The listing builds one solid part. Answer for the finished solid, in the listing's coordinates (mm). A direction names the side the tool comes from. Give positions to 0.01 mm unless a question says otherwise; leave off trailing zeros. Order: outer loops, then holes, each group sorted by start corner. A loop starts at its lowest first (then second) coordinate and runs counter-clockwise, first axis right, second up. Notation, with made-up numbers: M 5,15 L 14,15 A28 cw 14,52 Z; hole C -14,-24.75 d6. An arc over 180 degrees is marked long. Answer as a JSON object with one key per item and string values. Group by question number.
```python
from build123d import *

# Parameters (mm, degrees)
F1_DEPTH = 63.5
F2_DEPTH = 25.4
F3_DEPTH = 15.875


with BuildPart() as f1:
    # F0 (on Front) → F1 (new body, symmetric)
    with BuildSketch(Plane.XZ):
        Polygon((41.275, -9.525), (41.275, 9.525), (22.225, 9.525), (-41.275, 9.525), (-41.275, -9.525), align=None)
    extrude(amount=F1_DEPTH, both=True)

    # F0 (on Front) → F2 (join, symmetric)
    with BuildSketch(Plane.XZ):
        Polygon((41.275, -9.525), (41.275, 9.525), (22.225, 9.525), (-41.275, 9.525), (-41.275, -9.525), align=None)
        with BuildLine():
            Line((22.225, 9.525), (41.275, 9.525))
            Line((41.275, 9.525), (41.275, 36.094566609))
            ThreePointArc((41.275, 36.094566609), (37.2701177009, 42.5355625854), (35.2519640423, 49.8466888466))
            add(Edge.make_bspline(
                [(22.225, 41.2858579773), (27.1473848913, 43.2390175142), (31.5927512489, 45.8874426384), (35.2519640423, 49.8466888466)],
                knots=[68.7075286576, 68.7075286576, 68.7075286576, 68.7075286576, 85.3888938388, 85.3888938388, 85.3888938388, 85.3888938388], degree=3))
            Line((22.225, 41.2858579773), (22.225, 9.525))
        make_face()
        with BuildLine():
            Line((-41.275, 9.525), (22.225, 9.525))
            Line((22.225, 9.525), (22.225, 41.2858579773))
            add(Edge.make_bspline(
                [(-41.275, 9.525), (-26.416290782, 36.991388499), (1.9505861672, 33.2411468041), (22.225, 41.2858579773)],
                knots=[0, 0, 0, 0, 68.7075286576, 68.7075286576, 68.7075286576, 68.7075286576], degree=3))
        make_face()
        with BuildLine():
            ThreePointArc((35.2519640423, 49.8466888466), (37.2701177009, 42.5355625854), (41.275, 36.094566609))
            Line((41.275, 36.094566609), (41.275, 59.3244851528))
            add(Edge.make_bspline(
                [(35.2519640423, 49.8466888466), (37.6153515316, 52.4038598787), (39.6507933359, 55.5078428034), (41.275, 59.3244851528)],
                knots=[85.3888938388, 85.3888938388, 85.3888938388, 85.3888938388, 96.162940608, 96.162940608, 96.162940608, 96.162940608], degree=3))
        make_face()
        with BuildLine():
            Line((41.275, 59.3244851528), (41.275, 36.094566609))
            ThreePointArc((41.275, 36.094566609), (57.3677651162, 26.987491807), (75.5005331428, 30.6094559468))
            ThreePointArc((75.5005331428, 30.6094559468), (79.7565516079, 33.7035903942), (83.4994215816, 37.4020070167))
            Line((83.4994215816, 37.4020070167), (43.4881349932, 37.4020070167))
            Line((43.4881349932, 37.4020070167), (43.4881349932, 65.9770070167))
            add(Edge.make_bspline(
                [(41.275, 59.3244851528), (42.1309988934, 61.335954321), (42.872774659, 63.5453690941), (43.4881349932, 65.9770070167)],
                knots=[96.162940608, 96.162940608, 96.162940608, 96.162940608, 101.8411417359, 101.8411417359, 101.8411417359, 101.8411417359], degree=3))
        make_face()
        with BuildLine():
            Line((22.225, 60.325), (22.225, 41.2858579773))
            add(Edge.make_bspline(
                [(22.225, 41.2858579773), (27.1473848913, 43.2390175142), (31.5927512489, 45.8874426384), (35.2519640423, 49.8466888466)],
                knots=[68.7075286576, 68.7075286576, 68.7075286576, 68.7075286576, 85.3888938388, 85.3888938388, 85.3888938388, 85.3888938388], degree=3))
            ThreePointArc((35.2519640423, 49.8466888466), (53.353585698, 78.3955074484), (84.7937605886, 65.9770070167))
            Line((84.7937605886, 65.9770070167), (91.6146259472, 65.9770070167))
            ThreePointArc((91.6146259472, 65.9770070167), (54.3146372549, 95.1347162169), (22.225, 60.325))
        make_face()
        with BuildLine():
            Line((71.9847713728, 65.9770070167), (43.4881349932, 65.9770070167))
            Line((43.4881349932, 65.9770070167), (43.4881349932, 37.4020070167))
            Line((43.4881349932, 37.4020070167), (83.4994215816, 37.4020070167))
            ThreePointArc((83.4994215816, 37.4020070167), (90.7464246678, 50.7837278343), (91.6146259472, 65.9770070167))
            Line((91.6146259472, 65.9770070167), (84.7937605886, 65.9770070167))
            Line((84.7937605886, 65.9770070167), (71.9847713728, 65.9770070167))
        make_face()
        with BuildLine():
            ThreePointArc((91.6146259472, 65.9770070167), (90.7464246678, 50.7837278343), (83.4994215816, 37.4020070167))
            Line((83.4994215816, 37.4020070167), (94.2881349932, 37.4020070167))
            Line((94.2881349932, 37.4020070167), (94.2881349932, 65.9770070167))
            Line((94.2881349932, 65.9770070167), (91.6146259472, 65.9770070167))
        make_face()
    extrude(amount=F2_DEPTH, both=True)

    # F0 (on Front) + F2_face (on face) → F3 (join)
    with BuildSketch(Plane.XZ):
        Polygon((41.275, -9.525), (41.275, 9.525), (22.225, 9.525), (-41.275, 9.525), (-41.275, -9.525), align=None)
        with BuildLine():
            Line((22.225, 9.525), (41.275, 9.525))
            Line((41.275, 9.525), (41.275, 36.094566609))
            ThreePointArc((41.275, 36.094566609), (37.2701177009, 42.5355625854), (35.2519640423, 49.8466888466))
            add(Edge.make_bspline(
                [(22.225, 41.2858579773), (27.1473848913, 43.2390175142), (31.5927512489, 45.8874426384), (35.2519640423, 49.8466888466)],
                knots=[68.7075286576, 68.7075286576, 68.7075286576, 68.7075286576, 85.3888938388, 85.3888938388, 85.3888938388, 85.3888938388], degree=3))
            Line((22.225, 41.2858579773), (22.225, 9.525))
        make_face()
        with BuildLine():
            Line((-41.275, 9.525), (22.225, 9.525))
            Line((22.225, 9.525), (22.225, 41.2858579773))
            add(Edge.make_bspline(
                [(-41.275, 9.525), (-26.416290782, 36.991388499), (1.9505861672, 33.2411468041), (22.225, 41.2858579773)],
                knots=[0, 0, 0, 0, 68.7075286576, 68.7075286576, 68.7075286576, 68.7075286576], degree=3))
        make_face()
        with BuildLine():
            ThreePointArc((35.2519640423, 49.8466888466), (37.2701177009, 42.5355625854), (41.275, 36.094566609))
            Line((41.275, 36.094566609), (41.275, 59.3244851528))
            add(Edge.make_bspline(
                [(35.2519640423, 49.8466888466), (37.6153515316, 52.4038598787), (39.6507933359, 55.5078428034), (41.275, 59.3244851528)],
                knots=[85.3888938388, 85.3888938388, 85.3888938388, 85.3888938388, 96.162940608, 96.162940608, 96.162940608, 96.162940608], degree=3))
        make_face()
        with BuildLine():
            Line((41.275, 59.3244851528), (41.275, 36.094566609))
            ThreePointArc((41.275, 36.094566609), (57.3677651162, 26.987491807), (75.5005331428, 30.6094559468))
            ThreePointArc((75.5005331428, 30.6094559468), (79.7565516079, 33.7035903942), (83.4994215816, 37.4020070167))
            Line((83.4994215816, 37.4020070167), (43.4881349932, 37.4020070167))
            Line((43.4881349932, 37.4020070167), (43.4881349932, 65.9770070167))
            add(Edge.make_bspline(
                [(41.275, 59.3244851528), (42.1309988934, 61.335954321), (42.872774659, 63.5453690941), (43.4881349932, 65.9770070167)],
                knots=[96.162940608, 96.162940608, 96.162940608, 96.162940608, 101.8411417359, 101.8411417359, 101.8411417359, 101.8411417359], degree=3))
        make_face()
        with BuildLine():
            Line((22.225, 60.325), (22.225, 41.2858579773))
            add(Edge.make_bspline(
                [(22.225, 41.2858579773), (27.1473848913, 43.2390175142), (31.5927512489, 45.8874426384), (35.2519640423, 49.8466888466)],
                knots=[68.7075286576, 68.7075286576, 68.7075286576, 68.7075286576, 85.3888938388, 85.3888938388, 85.3888938388, 85.3888938388], degree=3))
            ThreePointArc((35.2519640423, 49.8466888466), (53.353585698, 78.3955074484), (84.7937605886, 65.9770070167))
            Line((84.7937605886, 65.9770070167), (91.6146259472, 65.9770070167))
            ThreePointArc((91.6146259472, 65.9770070167), (54.3146372549, 95.1347162169), (22.225, 60.325))
        make_face()
        with BuildLine():
            Line((71.9847713728, 65.9770070167), (43.4881349932, 65.9770070167))
            Line((43.4881349932, 65.9770070167), (43.4881349932, 37.4020070167))
            Line((43.4881349932, 37.4020070167), (83.4994215816, 37.4020070167))
            ThreePointArc((83.4994215816, 37.4020070167), (90.7464246678, 50.7837278343), (91.6146259472, 65.9770070167))
            Line((91.6146259472, 65.9770070167), (84.7937605886, 65.9770070167))
            Line((84.7937605886, 65.9770070167), (71.9847713728, 65.9770070167))
        make_face()
        with BuildLine():
            ThreePointArc((91.6146259472, 65.9770070167), (90.7464246678, 50.7837278343), (83.4994215816, 37.4020070167))
            Line((83.4994215816, 37.4020070167), (94.2881349932, 37.4020070167))
            Line((94.2881349932, 37.4020070167), (94.2881349932, 65.9770070167))
            Line((94.2881349932, 65.9770070167), (91.6146259472, 65.9770070167))
        make_face()
    with BuildSketch(Plane(origin=(39.5464553356, -25.4, 45.7929419382), x_dir=(1, 0, 0), z_dir=(0, -1, 0))):
        with BuildLine():
            Line((-80.8214553356, -36.2679419382), (1.7285446644, -36.2679419382))
            Line((1.7285446644, -36.2679419382), (1.7285446644, -9.6983753292))
            ThreePointArc((1.7285446644, -9.6983753292), (17.8213097807, -18.8054501311), (35.9540778072, -15.1834859914))
            ThreePointArc((35.9540778072, -15.1834859914), (40.2100962723, -12.089351544), (43.952966246, -8.3909349215))
            Line((43.952966246, -8.3909349215), (54.7416796576, -8.3909349215))
            Line((54.7416796576, -8.3909349215), (54.7416796576, 20.1840650785))
            Line((54.7416796576, 20.1840650785), (52.0681706117, 20.1840650785))
            ThreePointArc((52.0681706117, 20.1840650785), (14.7681819193, 49.3417742788), (-17.3214553356, 14.5320580618))
            Line((-17.3214553356, 14.5320580618), (-17.3214553356, -4.5070839609))
            add(Edge.make_bspline(
                [(-17.3214553356, -4.5070839609), (-37.5958691684, -12.5517951341), (-65.9627461175, -8.8015534392), (-80.8214553356, -36.2679419382)],
                knots=[129.2965536863, 129.2965536863, 129.2965536863, 129.2965536863, 198.004082344, 198.004082344, 198.004082344, 198.004082344], degree=3))
        make_face()
        with BuildLine():
            add(Edge.make_bspline(
                [(3.9416796576, 20.1840650785), (2.158709922, 13.1385397446), (-0.6855375098, 7.9586131706), (-4.2944912933, 4.0537469084)],
                knots=[96.162940608, 96.162940608, 96.162940608, 96.162940608, 112.6151885052, 112.6151885052, 112.6151885052, 112.6151885052], degree=3))
            ThreePointArc((-4.2944912933, 4.0537469084), (13.8071303624, 32.6025655102), (45.247305253, 20.1840650785))
            Line((45.247305253, 20.1840650785), (3.9416796576, 20.1840650785))
        make_face(mode=Mode.SUBTRACT)
    extrude(amount=F3_DEPTH)


solid = f1.part
```
Item 1: Section C-C (z = 5) is taken. Determine the outline of the cut face in (x, y) (3 decimals), and give its area (3 significant figures).
Item 2: Consider probe 1 along X at (y, z) = (-45, -1.5) (3 decimals); probe 2 along Z at (x, y) = (-25.5, -54) (3 decimals); probe 3 along Y at (x, z) = (52, 31) (3 decimals). Determine where each line is inside the solid, lowest interval first. Write a range as from..to.
Item 3: A tool of negligible diameter and unlimited length cuts with its end or side. For faces 4 (the flat face through (22.225, -8, 51)), 5 (the flat face through (41, 25.4, 43)), 6 (the flat face through (41.275, 1, 8)), 7 (the flat face through (1, -53, 9.525)), from which of +Z, -Z, +X, -X, +Y, -Y can it reach the whole face along a straight path? Write none if from no direction.
Item 4: Flat-ended cylindrical pins translate along their axes: P1, Ø12, axis at x = 43, y = 18.5, coming from the +Z side; P2, Ø12, axis at x = 47, z = 16, coming from the +Y side; P3, Ø5, axis at x = 28.5, z = 20.5, coming from the -Y side (3 decimals). Find the tip coordinate at first contact, or state that the pin passes through.
Item 5: Section B-B (y = 36) is taken. Determine the outline of the cut face in (x, z) (3 decimals).
Item 6: Section A-A (x = 78) is taken. Determine the outline of the cut face in (y, z) (3 decimals), and give its area (3 significant figures).
Item 7: Determine the mould class of faces 1 (the flat face through (64, -8, 65.977)), 2 (the flat face through (89, -7, 37.402)), 3 (the flat face through (41, -41.275, 43)) for opening direction Z: released by +Z, released by -Z, zero draft, split by the parting line, or undercut.
Values found:
{
 "1": {"outline": "M -41.275,-63.5 L 41.275,-63.5 L 41.275,63.5 L -41.275,63.5 Z", "area": "10,500 mm^2"},
 "2": {"probe 1": "x = -41.275..41.275", "probe 2": "z = -9.525..9.525", "probe 3": "y = -41.275..25.4"},
 "3": {"face 4": "+Z, -X, +Y, -Y", "face 5": "+Z, +X, -X, +Y", "face 6": "-Z, +Y, -Y", "face 7": "+Z, +X, -X, -Y"},
 "4": {"P1": "stops at z = 94.29", "P2": "stops at y = 25.4", "P3": "stops at y = -41.275"},
 "5": {"outline": "M -41.275,-9.525 L 41.275,-9.525 L 41.275,9.525 L -41.275,9.525 Z"},
 "6": {"outline": "M -41.275,32.307 L 25.4,32.307 L 25.4,65.977 L -41.275,65.977 Z; M -41.275,73.993 L 25.4,73.993 L 25.4,88.343 L -41.275,88.343 Z", "area": "3,200 mm^2"},
 "7": {"face 1": "undercut", "face 2": "released by -Z", "face 3": "zero draft"}
}
